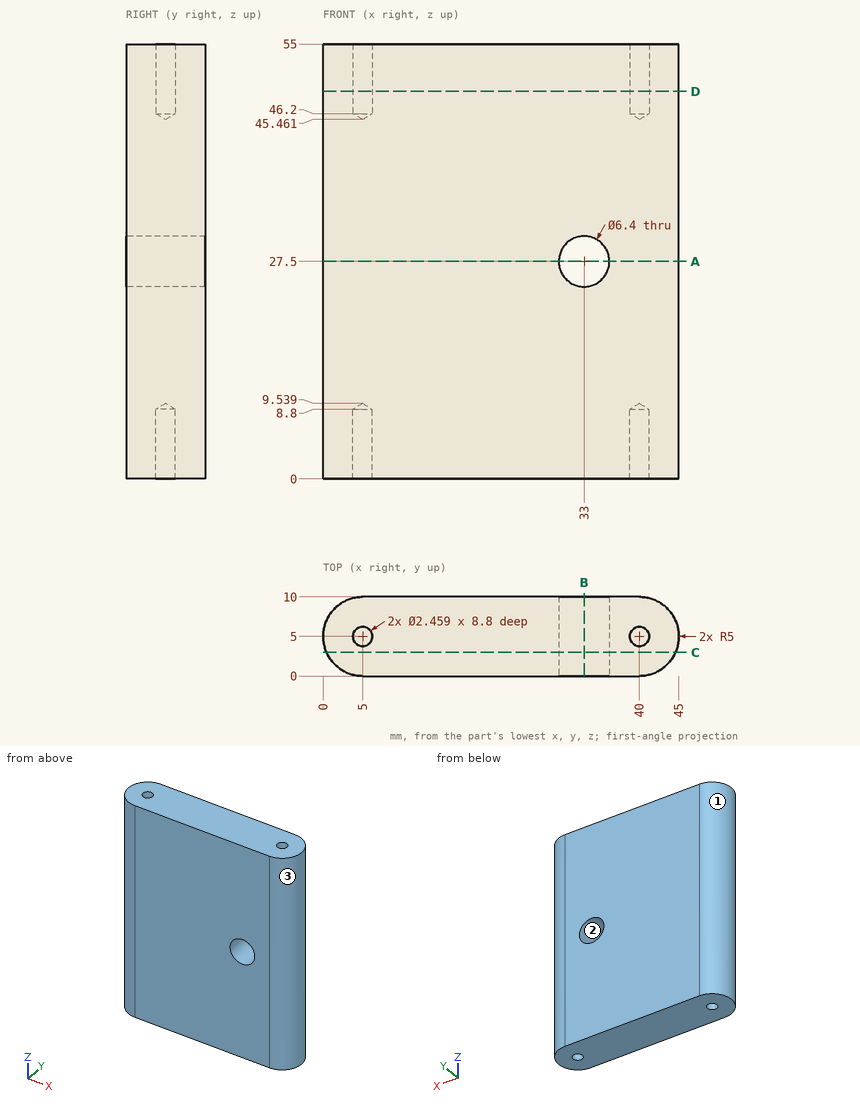
Geometry: see drawing. Coordinates: mm, zero at the bounding-box minimum. Round coordinates to 2 decimals unless told otherwise and drop trailing zeros. Loops run counter-clockwise (first coordinate to the right, second up) from the corner with the lowest first, then second, coordinate; pieces in that order, holes last. Notation, with made-up numbers: (55.25, 35) -> (101.25, 35) arc R28 cw to (101.25, 67) -> close; hole circle Ø2 at (-7.75, 20.25). An arc over 180 degrees is marked (long way). Write each question's results on one line, items separated by ' | '.
1. Ray query, line 1 (Y direction, x = 5, z = 52); line 2 (Z direction, x = 33, y = 7.75); line 3 (X direction, y = 3, z = 27.5). Return the intervals inside material, ascending. Write a range as from..to.
Geometry results:
line 1: 0..3.77, 6.23..10 | line 2: 0..24.3, 30.7..55 | line 3: 0.42..29.8, 36.2..44.58
2. Section C-C (y = 3). Return loops of the section in (x, z).
Geometry results:
outline: (0.42, 0) -> (44.58, 0) -> (44.58, 55) -> (0.42, 55) -> close; hole circle Ø6.4 at (33, 27.5)
3. Section B-B (x = 33). Return loops of the section in (y, z), and give its area (3 significant figures).
Geometry results:
outline: (0, 0) -> (10, 0) -> (10, 24.3) -> (0, 24.3) -> close; (0, 30.7) -> (10, 30.7) -> (10, 55) -> (0, 55) -> close | area: 486 mm2
4. Section A-A (z = 27.5). Return loops of the section in (x, y).
Geometry results:
outline: (5, 0) -> (29.8, 0) -> (29.8, 10) -> (5, 10) arc R5 ccw to start; (36.2, 0) -> (40, 0) arc R5 ccw to (40, 10) -> (36.2, 10) -> close
5. Section D-D (z = 49). Return loops of the section in (x, y).
Geometry results:
outline: (5, 0) -> (40, 0) arc R5 ccw to (40, 10) -> (5, 10) arc R5 ccw to start; hole circle Ø2.46 at (5, 5); hole circle Ø2.46 at (40, 5)
6. First-contact query: P1, Ø6, axis at x = 33, z = 27.5, coming from the -Y side; P2, Ø5, axis at y = 9, z = 17.5, coming from the +X side; P3, Ø1.5, axis at x = 5, y = 5, coming from the -Z side. Flat tips, straight axial feed; report the tip coordinate or a pass-through.
Geometry results:
P1: through | P2: x = 44.77 | P3: z = 9.09
7. Mould query, pull axis X, two halves, no side actions, for the marked faces 1, 2 and 3. Classes: +X half, -X half, draft (parallel to the pull), parting line (faces both ways), or undercut.
Geometry results:
face 1: -X half | face 2: undercut | face 3: +X half
